Input: part model. Units: mm. Frame: model coordinates. Round coordinates to 2 decimals unless told otherwise and drop trailing zeros. Loops run counter-clockwise (first coordinate to the right, second up) from the corner with the lowest first, then second, coordinate; pieces in that order, holes last. Notation, with made-up numbers: (32, 25.25) - (52, 25.25) arc R6 ccw to (52, 31.25) - close; hole circle Ø9 at (29.25, 66.5). An arc over 180 degrees is marked (long way). One line per question, with ' | ' between items. Start each with the question number.
Item 1: Material intervals for line 1 along X through (y, z) = (11.3, 1.3); line 2 along Y through (x, z) = (110.16, 0.8); line 3 along Y through (x, z) = (-110, 1.45), sorted ascending.
Item 2: Section D-D, the plane y = 38. Return loops of the section in (x, z).
Item 3: Section B-B, the plane y = 11.3. Return loops of the section in (x, z) (3 decimals).
Item 4: Section C-C, the plane x = -110. Return loops of the section in (y, z) (3 decimals), plus the area to 3 significant figures.
Item 5: Section A-A, the plane z = 1.6. Return loops of the section in (x, y), plus the area to 3 significant figures.
Item 6: Draft query along X for faces 1 (the face through (2, 38, 0)), 2 (the face through (-112.48, 12.08, 1.47)), 3 (the face through (-74.402, 56.843, 1.479)). Return one class per face: pulls with the +X half, pulls with the -X half, needs draft (parallel to the pull), parting line crosses it, or undercut.
```python
from build123d import *

# Parameters (mm, degrees)
Y_KSEKLIK_EKSTR_ZYON1_DEPTH                    = 3
M5_HELISARMAL_I_IN_Z_VANA_MATKAB_3_D           = 5.2
M5_HELISARMAL_I_IN_Z_VANA_MATKAB_3_DEPTH       = 18
M5_HELISARMAL_I_IN_Z_VANA_MATKAB_3_CSINK_D     = 5.25
M5_HELISARMAL_I_IN_Z_VANA_MATKAB_3_CSINK_ANGLE = 90
M5_HELISARMAL_I_IN_Z_VANA_MATKAB_3_TIP         = 1.562237609
M5_HELISARMAL_I_IN_Z_VANA_MATKAB_2_D           = 5.2
M5_HELISARMAL_I_IN_Z_VANA_MATKAB_2_DEPTH       = 18
M5_HELISARMAL_I_IN_Z_VANA_MATKAB_2_CSINK_D     = 5.25
M5_HELISARMAL_I_IN_Z_VANA_MATKAB_2_CSINK_ANGLE = 90
M5_HELISARMAL_I_IN_Z_VANA_MATKAB_2_TIP         = 1.562237609


with BuildPart() as part:
    # Çizim1 → Yükseklik-Ekstrüzyon1 (new body)
    with BuildSketch(Plane.XY):
        Polygon((150, 18), (150, 0), (-150, 0), (-150, 18), (3.342667003, 96.78849493), (69.768417769, 96.78849493), align=None)
    extrude(amount=Y_KSEKLIK_EKSTR_ZYON1_DEPTH)

    # M5 Helisarmal için Zıvana matkabı3
    with Locations(Plane.XY.offset(3)):
        with Locations((-110, 11.3), (110.16, 11.3)):
            CounterSinkHole(M5_HELISARMAL_I_IN_Z_VANA_MATKAB_3_D / 2, M5_HELISARMAL_I_IN_Z_VANA_MATKAB_3_CSINK_D / 2, depth=M5_HELISARMAL_I_IN_Z_VANA_MATKAB_3_DEPTH, counter_sink_angle=M5_HELISARMAL_I_IN_Z_VANA_MATKAB_3_CSINK_ANGLE)
            with Locations((0, 0, -(M5_HELISARMAL_I_IN_Z_VANA_MATKAB_3_DEPTH + M5_HELISARMAL_I_IN_Z_VANA_MATKAB_3_TIP / 2))):  # 118° drill point
                Cone(0, M5_HELISARMAL_I_IN_Z_VANA_MATKAB_3_D / 2, M5_HELISARMAL_I_IN_Z_VANA_MATKAB_3_TIP, mode=Mode.SUBTRACT)

    # M5 Helisarmal için Zıvana matkabı2
    with Locations(Plane.XY.offset(3)):
        with Locations((-110, 11.3), (110.16, 11.3)):
            CounterSinkHole(M5_HELISARMAL_I_IN_Z_VANA_MATKAB_2_D / 2, M5_HELISARMAL_I_IN_Z_VANA_MATKAB_2_CSINK_D / 2, depth=M5_HELISARMAL_I_IN_Z_VANA_MATKAB_2_DEPTH, counter_sink_angle=M5_HELISARMAL_I_IN_Z_VANA_MATKAB_2_CSINK_ANGLE)
            with Locations((0, 0, -(M5_HELISARMAL_I_IN_Z_VANA_MATKAB_2_DEPTH + M5_HELISARMAL_I_IN_Z_VANA_MATKAB_2_TIP / 2))):  # 118° drill point
                Cone(0, M5_HELISARMAL_I_IN_Z_VANA_MATKAB_2_D / 2, M5_HELISARMAL_I_IN_Z_VANA_MATKAB_2_TIP, mode=Mode.SUBTRACT)


solid = part.part
```
Return value:
1) line 1: -150 to -112.6, -107.4 to 107.56, 112.76 to 150 | line 2: 0 to 8.7, 13.9 to 57.12 | line 3: 0 to 8.7, 13.9 to 38.55
2) outline: (-111.07, 0) - (129.63, 0) - (129.63, 3) - (-111.07, 3) - close
3) outline: (-150, 0) - (-112.6, 0) - (-112.6, 2.975) - (-112.625, 3) - (-150, 3) - close; (-107.4, 0) - (107.56, 0) - (107.56, 2.975) - (107.535, 3) - (-107.375, 3) - (-107.4, 2.975) - close; (112.76, 0) - (150, 0) - (150, 3) - (112.785, 3) - (112.76, 2.975) - close
4) outline: (0, 0) - (8.7, 0) - (8.7, 2.975) - (8.675, 3) - (0, 3) - close; (13.9, 0) - (38.552, 0) - (38.552, 3) - (13.925, 3) - (13.9, 2.975) - close | area: 100 mm2
5) outline: (-150, 0) - (150, 0) - (150, 18) - (69.77, 96.79) - (3.34, 96.79) - (-150, 18) - close; hole circle Ø5.2 at (-110, 11.3); hole circle Ø5.2 at (110.16, 11.3) | area: 19,800 mm2
6) face 1: needs draft | face 2: undercut | face 3: pulls with the -X half
